Autodesk Inventor part; units mm, degrees
ref_plane "YZ Plane" through (0, 0, 0) normal (1, 0, 0) x (0, 1, 0)
ref_plane "XZ Plane" through (0, 0, 0) normal (0, 1, 0) x (-1, 0, 0)
ref_plane "XY Plane" through (0, 0, 0) normal (0, 0, 1) x (1, 0, 0)
sketch "草圖1" plane through (0, 0, 0) normal (1, 0, 0) x (0, 1, 0)
  line L0 (0, 9) -> (0, 9)
  line L1 (-3.125, 5.875) -> (-3.125, -5.875)
  line L2 (0, -9) -> (0, -9)
  line L3 (3.125, -5.875) -> (3.125, 5.875)
  line L4 (3.125, 9) -> (-3.125, -9) construction
  line L5 (-3.125, 9) -> (3.125, -9) construction
  circle A0 centre (0, 5.75) radius 1.6
  circle A1 centre (0, -5.75) radius 1.6
  arc A2 (0, -9) -> (3.125, -5.875) centre (0, -5.875) ccw
  arc A3 (-3.125, -5.875) -> (0, -9) centre (0, -5.875) ccw
  arc A4 (0, 9) -> (-3.125, 5.875) centre (0, 5.875) ccw
  arc A5 (3.125, 5.875) -> (0, 9) centre (0, 5.875) ccw
  point P0 (0, 0)
  point P1 (0, 0)
  point P2 (0, -9)
  point P3 (0, 9)
  dimension "d2" = 6.25
  dimension "d3" = 18
  dimension "d4" = 3.2
  dimension "d5" = 3.2
  dimension "d6" = 11.5
  dimension "d7" = 5.75
  dimension "d8" = 3.125
  dimension "d9" = 3.125
extrude "擠出1" add sketch "草圖1" along normal blind 1.8
sketch "草圖2" plane through (0, 0, 0) normal (0, 0, 1) x (1, 0, 0)
  line L0 (0, -3.125) -> (0, 3.125)
  line L1 (0, -3.125) -> (0, 7.375)
  line L2 (0, 7.375) -> (4, 7.375)
  line L3 (4, 7.375) -> (4, 0.875)
  line L4 (4, 0.875) -> (7.98, 0.875)
  line L5 (7.98, 0.875) -> (7.98, 7.375)
  line L6 (7.98, 7.375) -> (11.98, 7.375)
  line L7 (11.98, 7.375) -> (11.98, -3.125)
  line L8 (11.98, -3.125) -> (0, -3.125)
  point P0 (0, 0)
  dimension "d12" = 10.5
  dimension "d13" = 4
  dimension "d14" = 3.98
  dimension "d15" = 4
  dimension "d16" = 6.5
extrude "擠出2" add sketch "草圖2" along normal mid plane 6
properties part number "TP806 optic endstop"
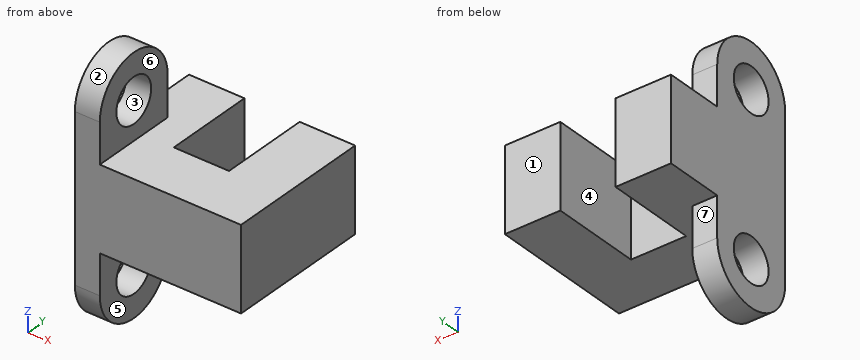
Work out the finished part from the listing and answer in its coordinate system (mm). Face numbers are marked on the shaded views. A direction names the side the tool comes from. Coordinates: 2 decimals unless noted, no trailing zeros. Write each loop counter-clockwise with the first axis right and the second up, starting at its lowest first coordinate (ties: lowest second). Pieces come first, ordered by that corner, then holes.
1. The part is cut by section B-B, the plane z = 0.75. Write down the section's boundary in (x, y) (3 decimals).
Results list:
outline: (0, -3.125) - (11.98, -3.125) - (11.98, 7.375) - (7.98, 7.375) - (7.98, 0.875) - (4, 0.875) - (4, 7.375) - (0, 7.375) - close
2. Flat-ended cylindrical pins translate along their axes: pin 1 (3.5 mm diameter, centred on y = 0, z = -5.75, fed in from +X); pin 2 (1.5 mm diameter, centred on x = 6, y = -0.5, fed in from -Z); pin 3 (2 mm diameter, centred on x = 6.5, z = -0.5, fed in from +Y) (3 decimals). Find the tip coordinate at first contact, or state that the pin passes through.
Results list:
pin 1: stops at x = 1.8
pin 2: stops at z = -3
pin 3: stops at y = 0.875
3. Consider line 1 along Z through (x, y) = (1, 0); line 2 along X through (y, z) = (3.75, -2.75); line 3 along Z through (x, y) = (0.5, 1.25). Determine where each line is inside the solid, lowest interval first.
Results list:
line 1: z = -9 to -7.35, -4.15 to 4.15, 7.35 to 9
line 2: x = 0 to 4, 7.98 to 11.98
line 3: z = -8.74 to -6.75, -4.75 to 4.75, 6.75 to 8.74
4. The part is cut by section C-C, the plane y = 0. Write down the section's boundary in (x, z).
Results list:
outline: (0, -9) - (1.8, -9) - (1.8, -7.35) - (0, -7.35) - close; (0, -4.15) - (1.8, -4.15) - (1.8, -3) - (11.98, -3) - (11.98, 3) - (1.8, 3) - (1.8, 4.15) - (0, 4.15) - close; (0, 7.35) - (1.8, 7.35) - (1.8, 9) - (0, 9) - close
5. The part is cut by section A-A, the plane y = 5. Write down the section's boundary in (x, z), and give its area (3 significant figures).
Results list:
outline: (0, -3) - (4, -3) - (4, 3) - (0, 3) - close; (7.98, -3) - (11.98, -3) - (11.98, 3) - (7.98, 3) - close
area: 48.0 mm2
6. For the marked faces 4, 5, 6 and 7, determine the directions among +Z, -Z, +X, -X, +Y, -Y from which every point of the face is accessible in a straight line to the end or side of a thin tool.
Results list:
face 4: +Z, -Z, +Y
face 5: -Z, +X, +Y, -Y
face 6: +Z, +X, +Y, -Y
face 7: -Z, +X, -X, +Y
7. For a pull along Z with two mould halves and no side action, classify the marked faces 1, 2 and 3 as +Z half, -Z half, draft (parallel to the pull), parting line (faces both ways), or undercut.
Results list:
face 1: draft
face 2: +Z half
face 3: undercut
8. The part is cut by section D-D, the plane z = 6.5. Write down the section's boundary in (x, y).
Results list:
outline: (0, -3.06) - (1.8, -3.06) - (1.8, -1.41) - (0, -1.41) - close; (0, 1.41) - (1.8, 1.41) - (1.8, 3.06) - (0, 3.06) - close
